Source: CAD feature listing. Evaluate the final solid. Frame: model axes, mm. Face numbers are marked on the shaded views. A direction names the side the tool comes from. Give positions to 0.01 mm unless a question says otherwise; leave off trailing zeros. Loops run counter-clockwise (first coordinate to the right, second up) from the corner with the lowest first, then second, coordinate; pieces in that order, holes last. Notation, with made-up numbers: (-26, -13.75) -> (11, -13.75) arc R15 cw to (11, 8.25) -> close; hole circle Ø4 at (3, -14). An arc over 180 degrees is marked (long way). Return JSON: item names as keys, results as strings. Group by question number.
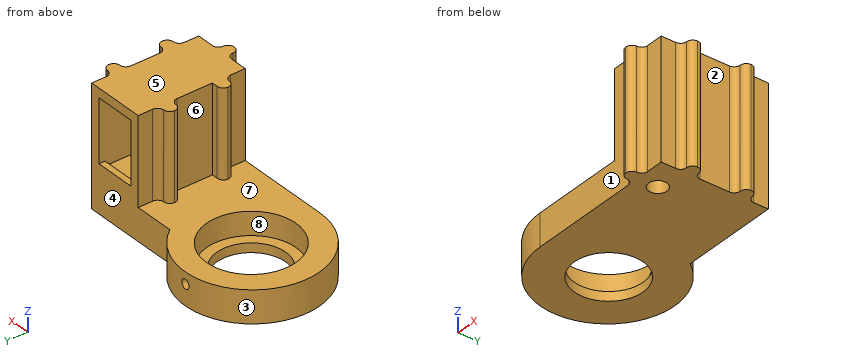
```python
from build123d import *

# Parameters (mm, degrees)
F0_R      = 22
F0_R_2    = 11.25
F1_DEPTH  = 10.5
F3_DEPTH  = 38.82
F4_R      = 14.625
F4_R_2    = 11.125
F5_DEPTH  = 7.5
F8_W      = 13.208
F8_H      = 20.32
F9_DEPTH  = 32.5
F10_R     = 3
F11_DEPTH = 15.4999664724
F12_W     = 13.208
F12_H     = 30.5
F13_DEPTH = 1.5
F14_W     = 13.208
F14_H     = 30.5
F15_DEPTH = 1
F16_W     = 30.8
F16_H     = 28.32
F17_DEPTH = 44.001
F18_W     = 4
F18_H     = 4
F19_DEPTH = 38.82
F20_R     = 1.99999
F7_R      = 1.5
F21_DEPTH = 10


# Not quite as in the source:
# - a fillet or chamfer is up to 0.001 mm smaller than in the source, because OpenCascade refuses the exact size
# - a feature names something its author has since deleted; it is built from what else it names


with BuildPart() as f1:
    # F0 (on Top) → F1 (new body)
    with BuildSketch(Plane.XY):
        Circle(F0_R)
        with Locations((-1.609e-06, 0.4174434871)):
            Circle(F0_R_2, mode=Mode.SUBTRACT)
    extrude(amount=F1_DEPTH)

    # F2 (on Top) → F3 (join)
    with BuildSketch(Plane.XY):
        with BuildLine():
            Line((0, -22), (50, -22))
            Line((50, -22), (50, 13))
            Line((50, 13), (17.7482393493, 13))
            ThreePointArc((17.7482393493, 13), (19.6214168703, -9.9498743711), (0, -22))
        make_face()
    extrude(amount=F3_DEPTH)

    # F4 (on face) → F5 (cut)
    with BuildSketch(Plane.XY.offset(10.5)):
        with Locations((-1.609e-06, 0.4174434871)):
            Circle(F4_R)
        with Locations((-1.609e-06, 0.4174434871)):
            Circle(F4_R_2, mode=Mode.SUBTRACT)
    extrude(amount=-F5_DEPTH, mode=Mode.SUBTRACT)

    # F8 (on face) → F9 (cut)
    with BuildSketch(Plane(origin=(0, 13, 0), x_dir=(-1, 0, 0), z_dir=(0, 1, 0))):
        with Locations((-40.396, 25.6599664724)):
            Rectangle(F8_W, F8_H)
    extrude(amount=-F9_DEPTH, mode=Mode.SUBTRACT)

    # F10 (on face) → F11 (cut, through all)
    with BuildSketch(Plane.XY.offset(15.4999664724)):
        with Locations((40.396, -15.5)):
            Circle(F10_R)
    extrude(amount=-F11_DEPTH, mode=Mode.SUBTRACT)

    # F12 (on face) → F13 (cut)
    with BuildSketch(Plane.XY.offset(15.4999664724)):
        with Locations((40.396, -4.25)):
            Rectangle(F12_W, F12_H)
    extrude(amount=-F13_DEPTH, mode=Mode.SUBTRACT)

    # F14 (on face) → F15 (cut)
    with BuildSketch(Plane(origin=(0, 0, 35.8199664724), x_dir=(1, 0, 0), z_dir=(0, 0, -1))):
        with Locations((40.396, 4.25)):
            Rectangle(F14_W, F14_H)
    extrude(amount=-F15_DEPTH, mode=Mode.SUBTRACT)

    # F16 (on face) → F17 (cut, through all)
    with BuildSketch(Plane.XZ.offset(22)):
        with Locations((15.4, 24.66)):
            Rectangle(F16_W, F16_H)
    extrude(amount=-F17_DEPTH, mode=Mode.SUBTRACT)

    # F18 (on face) → F19 (join, through all)
    with BuildSketch(Plane.XY.offset(38.82)):
        with Locations((52, 4.25)):
            Rectangle(F18_W, F18_H)
        with Locations((52, -13.25)):
            Rectangle(F18_W, F18_H)
        with Locations((28.8, -13.25)):
            Rectangle(F18_W, F18_H)
        with Locations((28.8, 4.25)):
            Rectangle(F18_W, F18_H)
        Polygon((40.4, -22), (38.4, -22), (38.4, -26), (42.4, -26), (42.4, -22), align=None)
    extrude(amount=-F19_DEPTH)

    # F20 (radius 2 in the source; OpenCascade refuses exactly that, so slightly less here)
    f20_edges = [f1.edges().sort_by_distance(p)[0] for p in [
        (42.4, -26, 19.41),
        (38.4, -26, 19.41),
        (42.4, -22, 19.41),
        (50, -15.25, 19.41),
        (54, -15.25, 19.41),
        (54, -11.25, 19.41),
        (50, 2.25, 19.41),
        (54, 2.25, 19.41),
        (54, 6.25, 19.41),
        (26.8, 2.25, 24.66),
        (26.8, -15.25, 24.66),
        (50, -11.25, 19.41),
        (50, 6.25, 19.41),
        (38.4, -22, 19.41),
        (26.8, -11.25, 24.66),
        (26.8, 6.25, 24.66),
        (30.8, 6.25, 24.66),
        (30.8, 2.25, 24.66),
        (30.8, -15.25, 24.66),
    ]]
    fillet(f20_edges, radius=F20_R)

    # F7 (on offset) → F21 (cut)
    with BuildSketch(Plane.XZ.offset(-22)):
        with Locations((0, 6.75)):
            Circle(F7_R)
    extrude(amount=F21_DEPTH, mode=Mode.SUBTRACT)


solid = f1.part
```
1) Material intervals for line 1 (X direction, y = -6, z = 17.5); line 2 (Z direction, x = 0, y = 17.5); line 3 (Z direction, x = 0.5, y = 13), sorted ascending.
2) Reachability of the marked faces 1, 2, 3, 4 and 5 from +Z, -Z, +X, -X, +Y, -Y: full face, straight path, thin tool, end or side. Return the list, or none.
3) Cut plane A-A on y = 10. Return loops of the section in (x, z), then the cut area to 3 significant figures.
4) Cut plane B-B on x = 3.5. Return loops of the section in (y, z).
5) Cut plane D-D on x = 12.5. Return loops of the section in (y, z), then the cut area to 3 significant figures.
6) Contact query for flat-ended pins moving along their axis: P1, Ø4, axis at y = 11, z = 18, coming from the -X side; P2, Ø10.5, axis at x = 40.5, z = 29.5, coming from the +Y side; P3, Ø11, axis at x = 22, z = 13.5, coming from the -Y side. Output: stop coordinate, or through.
7) Mould query, pull axis X, two halves, no side actions, for the marked faces 6, 7 and 8. Classes: released by +X, released by -X, zero draft, split by the parting line, or undercut.
Calculated:
{
 "1": {"line 1": "30.8 to 33.79, 47 to 50", "line 2": "0 to 5.25, 8.25 to 10.5", "line 3": "0 to 3"},
 "2": {"face 1": "+Z, -Z, -X, -Y", "face 2": "+Z, -Z, +X", "face 3": "+Z, -Z", "face 4": "+Z, -Z, +X, +Y", "face 5": "+Z, +X, -X, +Y, -Y"},
 "3": {"outline": "(-19.6, 0) -> (-5.89, 0) -> (-5.89, 3) -> (-11.05, 3) -> (-11.05, 10.5) -> (-19.6, 10.5) -> close; (5.89, 0) -> (50, 0) -> (50, 38.82) -> (30.8, 38.82) -> (30.8, 10.5) -> (11.05, 10.5) -> (11.05, 3) -> (5.89, 3) -> close; hole (33.79, 14) -> (47, 14) -> (47, 36.82) -> (33.79, 36.82) -> close", "area": "772 mm2"},
 "4": {"outline": "(-22, 0) -> (-10.27, 0) -> (-10.27, 3) -> (-13.78, 3) -> (-13.78, 10.5) -> (-22, 10.5) -> close; (11.11, 0) -> (21.72, 0) -> (21.72, 10.5) -> (14.62, 10.5) -> (14.62, 3) -> (11.11, 3) -> close"},
 "5": {"outline": "(-22, 0) -> (18.1, 0) -> (18.1, 10.5) -> (8.01, 10.5) -> (8.01, 3) -> (-7.17, 3) -> (-7.17, 10.5) -> (-22, 10.5) -> close", "area": "307 mm2"},
 "6": {"P1": "x = 30.8", "P2": "y = -19.5", "P3": "y = -22"},
 "7": {"face 6": "released by -X", "face 7": "zero draft", "face 8": "undercut"}
}
